```python
from build123d import *

# Parameters (mm, degrees)
F0_W     = 10
F0_H     = 10
F1_DEPTH = 75
F2_R     = 2
F3_DEPTH = 9


with BuildPart() as f1:
    # F0 (on Front) → F1 (new body)
    with BuildSketch(Plane.XZ):
        with Locations((0.008259, 0)):
            Rectangle(F0_W, F0_H)
    extrude(amount=F1_DEPTH)

    # F2 (on face) → F3 (join)
    with BuildSketch(Plane.XZ.offset(75)):
        Circle(F2_R)
    extrude(amount=F3_DEPTH)


solid = f1.part
```
Geometry: final body of the model. Coordinates: model frame, mm. A direction names the side the tool comes from. Give positions to 0.01 mm unless a question says otherwise; leave off trailing zeros. Loops run counter-clockwise (first coordinate to the right, second up) from the corner with the lowest first, then second, coordinate; pieces in that order, holes last. Notation, with made-up numbers: (-26.5, 15) -> (25.5, 15) arc R21 cw to (25.5, 29) -> close; hole circle Ø3 at (32.5, 62.5). An arc over 180 degrees is marked (long way). Use CSV: the item, a comma, the result in double quotes.
(1) Cut plane A-A (x = 0). Output: boundary loops of the cut face in (y, z).
From the geometry:
outline,"(-84, -2) -> (-75, -2) -> (-75, -5) -> (0, -5) -> (0, 5) -> (-75, 5) -> (-75, 2) -> (-84, 2) -> close"
(2) Cut plane C-C (y = -77). Output: boundary loops of the cut face in (x, z).
From the geometry:
outline,"circle Ø4 at (0, 0)"
(3) Cut plane B-B (z = 0). Output: boundary loops of the cut face in (x, y), plus the area to 3 significant figures.
From the geometry:
outline,"(-4.99, -75) -> (-2, -75) -> (-2, -84) -> (2, -84) -> (2, -75) -> (5.01, -75) -> (5.01, 0) -> (-4.99, 0) -> close"
area,"786 mm^2"
(4) Ray query, line 1 along Y through (x, z) = (-1.5, -3.25); line 2 along Z through (x, y) = (1.5, -79). Return the intervals inside material, ascending. Write a range as [from, to].
From the geometry:
line 1,"[-75, 0]"
line 2,"[-1.32, 1.32]"
(5) Access query for faces 1 (the face through (0, -37, -5)), 2 (the face through (0, -79, -2)). Directions: +Z, -Z, +X, -X, +Y, -Y. A direction counts if a zero-diameter tool reaches every point of the face in a straight line with its end or side. Return the directions, or none.
From the geometry:
face 1,"-Z, +X, -X, +Y, -Y"
face 2,"-Y"
(6) Cut plane D-D (z = 4). Output: boundary loops of the cut face in (x, y), plus the area to 3 significant figures.
From the geometry:
outline,"(-4.99, -75) -> (5.01, -75) -> (5.01, 0) -> (-4.99, 0) -> close"
area,"750 mm^2"
